```python
from build123d import *

# Parameters (mm, degrees)
BOSS_EXTRU_1_DEPTH      = 254.666666667
ESQUISSE4_R             = 54.250129783
ESQUISSE4_R_2           = 27.5
ENL_V_MAT_EXTRU_1_DEPTH = 266.174026394
ESQUISSE5_R             = 10
ESQUISSE5_R_2           = 3
ESQUISSE5_W             = 1.7
ESQUISSE5_H             = 10
ENL_V_MAT_EXTRU_2_DEPTH = 258.315177949


with BuildPart() as part:
    # Esquisse1 → Boss.-Extru.1 (new body)
    with BuildSketch(Plane.XY):
        with BuildLine():
            Line((-18, -51.176914536), (-18, -48.176914536))
            ThreePointArc((-18, -48.176914536), (-9.5, -16.454482672), (-32.722431864, -39.676914536))
            Line((-32.722431864, -39.676914536), (-35.320508076, -41.176914536))
            ThreePointArc((-35.320508076, -41.176914536), (-37.98683472, -30.451354144), (-34.549834435, -19.947356212))
            ThreePointArc((-34.549834435, -19.947356212), (-45.365063628, -17.671886805), (-53.320508076, -10))
            Line((-53.320508076, -10), (-50.722431864, -8.5))
            ThreePointArc((-50.722431864, -8.5), (-19, 0), (-50.722431864, 8.5))
            Line((-50.722431864, 8.5), (-53.320508076, 10))
            ThreePointArc((-53.320508076, 10), (-45.365063628, 17.671886805), (-34.549834435, 19.947356212))
            ThreePointArc((-34.549834435, 19.947356212), (-37.98683472, 30.451354144), (-35.320508076, 41.176914536))
            Line((-35.320508076, 41.176914536), (-32.722431864, 39.676914536))
            ThreePointArc((-32.722431864, 39.676914536), (-9.5, 16.454482672), (-18, 48.176914536))
            Line((-18, 48.176914536), (-18, 51.176914536))
            ThreePointArc((-18, 51.176914536), (-7.378228908, 48.123240948), (0, 39.894712423))
            ThreePointArc((0, 39.894712423), (7.378228908, 48.123240948), (18, 51.176914536))
            Line((18, 51.176914536), (18, 48.176914536))
            ThreePointArc((18, 48.176914536), (9.5, 16.454482672), (32.722431864, 39.676914536))
            Line((32.722431864, 39.676914536), (35.320508076, 41.176914536))
            ThreePointArc((35.320508076, 41.176914536), (37.98683472, 30.451354144), (34.549834435, 19.947356212))
            ThreePointArc((34.549834435, 19.947356212), (45.365063628, 17.671886805), (53.320508076, 10))
            Line((53.320508076, 10), (50.722431864, 8.5))
            ThreePointArc((50.722431864, 8.5), (19, 0), (50.722431864, -8.5))
            Line((50.722431864, -8.5), (53.320508076, -10))
            ThreePointArc((53.320508076, -10), (45.365063628, -17.671886805), (34.549834435, -19.947356212))
            ThreePointArc((34.549834435, -19.947356212), (37.98683472, -30.451354144), (35.320508076, -41.176914536))
            Line((35.320508076, -41.176914536), (32.722431864, -39.676914536))
            ThreePointArc((32.722431864, -39.676914536), (9.5, -16.454482672), (18, -48.176914536))
            Line((18, -48.176914536), (18, -51.176914536))
            ThreePointArc((18, -51.176914536), (7.378228908, -48.123240948), (0, -39.894712423))
            ThreePointArc((0, -39.894712423), (-7.378228908, -48.123240948), (-18, -51.176914536))
        make_face()
    extrude(amount=BOSS_EXTRU_1_DEPTH)

    # Esquisse4 → Enlèv. mat.-Extru.1 (cut, through all)
    with BuildSketch(Plane.XY.offset(254.666666667)):
        Circle(ESQUISSE4_R)
        Circle(ESQUISSE4_R_2, mode=Mode.SUBTRACT)
    extrude(amount=-ENL_V_MAT_EXTRU_1_DEPTH, mode=Mode.SUBTRACT)

    # Esquisse5 → Enlèv. mat.-Extru.2 (cut, through all)
    with BuildSketch(Plane.XY.offset(254.666666667)):
        Circle(ESQUISSE5_R)
        with Locations((0, 15)):
            Circle(ESQUISSE5_R_2)
        with Locations((12.990381057, 7.5)):
            Circle(ESQUISSE5_R_2)
        with Locations((12.990381057, -7.5)):
            Circle(ESQUISSE5_R_2)
        with Locations((0, -15)):
            Circle(ESQUISSE5_R_2)
        with Locations((-12.990381057, 7.5)):
            Circle(ESQUISSE5_R_2)
        Polygon((14.206088614, -14.605667257), (5.545834576, -19.605667257), (4.695834576, -18.13342407), (13.356088614, -13.13342407), align=None)
        Polygon((18.051923191, 5), (19.751923191, 5), (19.751923191, -5), (18.051923191, -5), (18.051923191, -1.5), (14.051923191, -1.5), (14.051923191, 1.5), (18.051923191, 1.5), align=None)
        Polygon((-5.545834576, -19.605667257), (-14.206088614, -14.605667257), (-13.356088614, -13.13342407), (-4.695834576, -18.13342407), align=None)
        with Locations((-18.901923191, 0)):
            Rectangle(ESQUISSE5_W, ESQUISSE5_H)
        Polygon((-14.206088614, 14.605667257), (-5.545834576, 19.605667257), (-4.695834576, 18.13342407), (-13.356088614, 13.13342407), align=None)
        Polygon((5.545834576, 19.605667257), (14.206088614, 14.605667257), (13.356088614, 13.13342407), (4.695834576, 18.13342407), align=None)
    extrude(amount=-ENL_V_MAT_EXTRU_2_DEPTH, mode=Mode.SUBTRACT)


solid = part.part
```
Work out the finished part from the listing and answer in its coordinate system (mm). A direction names the side the tool comes from. Give positions to 0.01 mm unless a question says otherwise; leave off trailing zeros. Loops run counter-clockwise (first coordinate to the right, second up) from the corner with the lowest first, then second, coordinate; pieces in that order, holes last. Notation, with made-up numbers: (-8.75, 26) - (48.25, 26) arc R9 ccw to (48.25, 31) - close; hole circle Ø3 at (0, -5). An arc over 180 degrees is marked (long way). One line per question, with ' | ' between items.
(1) Straight lines are drawn through the part: probe 1 along Y at (x, z) = (15, 204.5); probe 2 along Y at (x, z) = (1, 230); probe 3 along X at (y, z) = (7, 153). For each, find the intervals that lie inside material, in ascending order.
Recorded:
probe 1: y = -14.44 to -9.73, -5.27 to -1.5, 1.5 to 5.27, 9.73 to 14.44 | probe 2: y = -27.48 to -17.83, -12.17 to -9.95, 9.95 to 12.17, 17.83 to 27.48 | probe 3: x = -20.51 to -15.95, -10.03 to -7.14, 7.14 to 10.03, 15.95 to 20.51
(2) The part is cut by section A-A (y = 7.5). Write down the section's boundary in (x, z).
Recorded:
outline: (-20.74, 0) - (-15.99, 0) - (-15.99, 254.67) - (-20.74, 254.67) - close; (-9.99, 0) - (-6.61, 0) - (-6.61, 254.67) - (-9.99, 254.67) - close; (6.61, 0) - (9.99, 0) - (9.99, 254.67) - (6.61, 254.67) - close; (15.99, 0) - (20.74, 0) - (20.74, 254.67) - (15.99, 254.67) - close
(3) The part is cut by section B-B (z = 235). Count the separate pieces of the cut face and the enclosed holes in it, then the cut area to 3 significant figures.
Recorded:
separate pieces: 1 | enclosed holes: 6 | area: 962 mm²
(4) A tool of negligible diameter and unlimited length cuts with its end or side. For faces 1 (the face through (16, -1.5, 129)), 2 (the face through (-21.59, 9.02, 125.55)), 3 (the face through (2.927, 23.316, 125.551)), from which of +Z, -Z, +X, -X, +Y, -Y can it reach the whole face along a straight path? Write none if from no direction.
Recorded:
face 1: +Z, -Z, +X | face 2: +Z, -Z, -X | face 3: +Z, -Z, +X, +Y
(5) The mould has two halves that part along X. Classify faces 4 (the face through (2.985, -23.204, 125.551)), 5 (the face through (9.087, 15.598, 129.116)), 6 (the face through (-0.65, -17.93, 129.12)), 7 (the face through (-2.985, 23.204, 125.551)): +X half, -X half, draft (parallel to the pull), parting line (faces both ways), or undercut.
Recorded:
face 4: +X half | face 5: undercut | face 6: undercut | face 7: -X half
(6) Each of these flat-tipped pins is pushed along its axis until it touches: pin 1 Ø1 at (y, z) = (-2.5, 112.5) entering from +X; pin 2 Ø3 at (x, z) = (-7, 186.5) entering from -Y; pin 3 Ø4.5 at (x, z) = (16.5, 68.5) entering from +Y. Where does it stop, or does it pass through?
Recorded:
pin 1: stops at x = 18.05 | pin 2: stops at y = -19.66 | pin 3: stops at y = 14.6
